Verification items for the finished model (mm, model axes). Face numbers are marked on the shaded views. A direction names the side the tool comes from. Give positions to 0.01 mm unless a question says otherwise; leave off trailing zeros. Loops run counter-clockwise (first coordinate to the right, second up) from the corner with the lowest first, then second, coordinate; pieces in that order, holes last. Notation, with made-up numbers: (78.5, -11) - (87.5, -11) arc R28 cw to (87.5, 19) - close; hole circle Ø2 at (-30, 0). An arc over 180 degrees is marked (long way). One line per item, written item: value. Start each with the question number.
1. Access from +Z, -Z, +X, -X, +Y, -Y to the whole of each face (thin tool, end or side, straight path). Record for the marked faces 5 and 6.
2. Sectioned sample at A-A (x = 0.75). Record the cut outline in (y, z), plus the area to 3 significant figures.
3. Scan lines: L1, parallel to Y at x = 1.5, z = -1.75; L2, parallel to Y at x = 6.75, z = -2; L3, parallel to Z at x = 5.5, y = -0.9. Record each from-to range of solid material in increasing order. Write a range as [from, to].
4. Gauge pin test, flat ends, axial feed: pin 1 (3 mm diameter, centred on x = 4.5, z = -3.5, fed in from -Y); pin 2 (2 mm diameter, centred on y = 1.5, z = -2.5, fed in from +X); pin 3 (1 mm diameter, centred on x = 3.5, y = -1, fed in from +Z). Record the tip position at first contact, or that the pin passes through.
5. Mould release check, pull along Z, two halves, no side actions. Record for the marked faces 1, 2, 3 and 4: pulls with the +Z half, pulls with the -Z half, needs draft (parallel to the pull), parting line crosses it, or undercut.
6. Sectioned sample at C-C (z = -6.75). Record the cut outline in (x, y).
7. Sectioned sample at B-B (y = 1.6). Record the cut outline in (x, z).
from build123d import *

# Parameters (mm, degrees)
SKETCH1_W               = 8
SKETCH1_H               = 8
BOSS_EXTRUDE1_DEPTH     = 3
CUT_EXTRUDE1_DEPTH      = 12.704699911
CUT_EXTRUDE1_DEPTH_BACK = 12.704699911
CUT_EXTRUDE2_DEPTH      = 11
SKETCH4_R               = 1.75
CUT_EXTRUDE3_DEPTH      = 0.4
SKETCH5_W               = 8
SKETCH5_H               = 1
BOSS_EXTRUDE2_DEPTH     = 2
FILLET1_R               = 4
CUT_EXTRUDE4_DEPTH      = 0.4
CUT_EXTRUDE5_DEPTH      = 0.5


with BuildPart() as part:
    # Sketch1 → Boss-Extrude1 (new body)
    with BuildSketch(Plane(origin=(0, 0, 0), x_dir=(1, 0, 0), z_dir=(0, 1, 0))):
        with Locations((4, 4)):
            Rectangle(SKETCH1_W, SKETCH1_H)
    extrude(amount=BOSS_EXTRUDE1_DEPTH)

    # Sketch2 → Cut-Extrude1 (cut, two sides: drawn at the far end of the back side and taken through both)
    with BuildSketch(Plane.XY.offset(-CUT_EXTRUDE1_DEPTH_BACK)):
        Polygon((0, 0), (0.6, 3), (0, 3), align=None)
        Polygon((8, 0), (7.4, 3), (8, 3), align=None)
    extrude(amount=CUT_EXTRUDE1_DEPTH + CUT_EXTRUDE1_DEPTH_BACK, mode=Mode.SUBTRACT)

    # Sketch3 → Cut-Extrude2 (cut)
    with BuildSketch(Plane(origin=(0, 0, 0), x_dir=(0, 0, -1), z_dir=(1, 0, 0))):
        Polygon((0, 0), (0.6, 3), (0, 3), align=None)
        Polygon((8, 3), (7.4, 3), (8, 0), align=None)
    extrude(amount=CUT_EXTRUDE2_DEPTH, mode=Mode.SUBTRACT)

    # Sketch4 → Cut-Extrude3 (cut)
    with BuildSketch(Plane.XZ):
        with Locations(Location((4, -3.75, 0), (0, 0, 270))):
            Circle(SKETCH4_R)
    extrude(amount=-CUT_EXTRUDE3_DEPTH, mode=Mode.SUBTRACT)

    # Sketch5 → Boss-Extrude2 (add)
    with BuildSketch(Plane.XZ):
        with Locations((4, -7.5)):
            Rectangle(SKETCH5_W, SKETCH5_H)
    extrude(amount=BOSS_EXTRUDE2_DEPTH)

    # Fillet1
    # the kernel refuses this fillet: 4 mm, written as the material it takes off along each edge
    with BuildSketch(Plane(origin=(8, -2, -16.660254038), x_dir=(0, 1, 0), z_dir=(0, 0, 1)), Plane(origin=(0, -2, 1.660254038), x_dir=(0, 1, 0), z_dir=(0, 0, -1))) as fillet1_piece_1:
        with BuildLine():
            CenterArc((4, 3.464101615), FILLET1_R, 180, 60)
            Line((0, 3.464101615), (-0.08, 3.464101615))
            Line((-0.08, 3.464101615), (-0.08, 0))
            Line((-0.08, 0), (0, -0.08))
            ThreePointArc((0, -0.08), (1, -0.08), (1.96, -0.069282032))
            Line((1.96, -0.069282032), (2, 0))
        make_face()
    extrude(amount=18.320508076, mode=Mode.SUBTRACT)

    # Sketch6 → Cut-Extrude4 (cut)
    with BuildSketch(Plane(origin=(0, 3, 0), x_dir=(1, 0, 0), z_dir=(0, 1, 0))):
        with BuildLine():
            add(Edge.make_bspline(
                [(5.284087955, 2.773445367), (5.333545491, 2.739545524), (5.432652736, 2.671614118), (5.590291823, 2.583736248), (5.752942084, 2.503846486), (5.865979951, 2.460876102), (5.92270975, 2.439310751)],
                knots=[0, 0, 0, 0, 0.994855506, 1.99357661, 2.993045438, 4, 4, 4, 4], degree=3))
            Line((5.92270975, 2.439310751), (5.628639237, 1.875208187))
            add(Edge.make_bspline(
                [(5.628639237, 1.875208187), (5.568520037, 1.893818156), (5.447325875, 1.93133395), (5.332925255, 1.986187111), (5.275273852, 2.013829982)],
                knots=[0, 0, 0, 0, 0.992113803, 2, 2, 2, 2], degree=3))
            add(Edge.make_bspline(
                [(5.275273852, 2.013829982), (5.26961656, 2.016684314), (5.253233801, 2.024950075), (5.223476786, 2.045298413), (5.178074812, 2.072724498), (5.118973761, 2.11071311), (5.045578888, 2.157800121), (4.95765273, 2.213934729), (4.856407872, 2.280704114), (4.783596416, 2.327731001), (4.744825134, 2.35277229)],
                knots=[0, 0, 0, 0, 0.241377655, 0.698997227, 1.371388316, 2.263975901, 3.376788369, 4.695767198, 6.240533187, 8, 8, 8, 8], degree=3))
            add(Edge.make_bspline(
                [(4.744825134, 2.35277229), (4.712670389, 2.339001865), (4.648050063, 2.311327899), (4.547788838, 2.27725121), (4.444978029, 2.248544986), (4.339982896, 2.224200245), (4.232359046, 2.206111381), (4.122258624, 2.192239309), (4.00937299, 2.18410397), (3.933139287, 2.183304154), (3.894664878, 2.182900495)],
                knots=[0, 0, 0, 0, 0.961025642, 1.931341354, 2.907359807, 3.893838693, 4.891829695, 5.905170566, 6.942759923, 8, 8, 8, 8], degree=3))
            add(Edge.make_bspline(
                [(3.894664878, 2.182900495), (3.821683976, 2.184676763), (3.679027131, 2.188148859), (3.471015208, 2.212756542), (3.275562804, 2.255408477), (3.091812023, 2.313667662), (2.920867424, 2.390147666), (2.761229426, 2.482594503), (2.615108223, 2.593406711), (2.480490537, 2.71918809), (2.361392609, 2.861354588), (2.257130725, 3.017424584), (2.168806746, 3.186880722), (2.097587685, 3.370615377), (2.041301668, 3.567142879), (2.002926315, 3.777850586), (1.978227581, 4.001488849), (1.975427333, 4.155321196), (1.973991801, 4.234182546)],
                knots=[0, 0, 0, 0, 1.098101164, 2.146474535, 3.146072545, 4.104420533, 5.041773038, 5.958565538, 6.874115049, 7.795336865, 8.725215067, 9.658214839, 10.614563411, 11.594512188, 12.618591104, 13.685899083, 14.813688224, 16, 16, 16, 16], degree=3))
            add(Edge.make_bspline(
                [(1.973991801, 4.234182546), (1.97543059, 4.313040679), (1.978227497, 4.466335509), (2.002757559, 4.689542909), (2.042412611, 4.899497801), (2.098124704, 5.096337583), (2.170410456, 5.279545107), (2.259079723, 5.449017762), (2.363505524, 5.605417057), (2.484015277, 5.747270094), (2.617919267, 5.874338646), (2.764464989, 5.984327234), (2.9219486, 6.078236158), (3.090996271, 6.154643933), (3.272074664, 6.212871015), (3.463805003, 6.255387163), (3.667248709, 6.280295733), (3.806454886, 6.283712517), (3.877837955, 6.285464598)],
                knots=[0, 0, 0, 0, 1.193283781, 2.319662245, 3.393996131, 4.424093603, 5.411284417, 6.369670503, 7.313761776, 8.251713527, 9.181123148, 10.102053383, 11.01932051, 11.951118596, 12.903560284, 13.893239571, 14.919681386, 16, 16, 16, 16], degree=3))
            add(Edge.make_bspline(
                [(3.877837955, 6.285464598), (3.948708316, 6.284176334), (4.086935049, 6.281663683), (4.288489067, 6.254790298), (4.478939684, 6.214016744), (4.658513444, 6.155241629), (4.826290277, 6.078911265), (4.983143341, 5.98623667), (5.128157857, 5.876434989), (5.26137487, 5.750578969), (5.380523981, 5.609215368), (5.486073462, 5.454669187), (5.572731816, 5.285035211), (5.645736122, 5.103191508), (5.700157026, 4.90736457), (5.740330715, 4.69867705), (5.764520815, 4.476471411), (5.76739165, 4.323719862), (5.768863596, 4.245400495)],
                knots=[0, 0, 0, 0, 1.078752742, 2.104017338, 3.091035458, 4.041673215, 4.975566109, 5.892967701, 6.810684895, 7.740128604, 8.678185021, 9.621404646, 10.583875016, 11.573429805, 12.6009998, 13.674031063, 14.80742018, 16, 16, 16, 16], degree=3))
            add(Edge.make_bspline(
                [(5.768863596, 4.245400495), (5.767275795, 4.16278925), (5.764189157, 4.002195454), (5.737326284, 3.768977018), (5.693780668, 3.550562854), (5.648918616, 3.41330904), (5.627036673, 3.346362034)],
                knots=[0, 0, 0, 0, 1.083667057, 2.106616435, 3.076482036, 4, 4, 4, 4], degree=3))
            add(Edge.make_bspline(
                [(5.627036673, 3.346362034), (5.607421404, 3.297050064), (5.567517691, 3.196733787), (5.488642668, 3.051933408), (5.394797316, 2.909076479), (5.321514211, 2.819296637), (5.284087955, 2.773445367)],
                knots=[0, 0, 0, 0, 0.948216854, 1.928975575, 2.942311585, 4, 4, 4, 4], degree=3))
        make_face()
        with BuildLine():
            add(Edge.make_bspline(
                [(4.642261032, 3.185304341), (4.671182259, 3.216922768), (4.72909393, 3.280235293), (4.800707281, 3.388678336), (4.863230922, 3.50497094), (4.912388312, 3.632014464), (4.951923574, 3.76787431), (4.97951585, 3.913560578), (4.996652709, 4.068707035), (4.998621406, 4.175375245), (4.999632827, 4.230176136)],
                knots=[0, 0, 0, 0, 0.906820982, 1.815812261, 2.745108282, 3.70056618, 4.696560745, 5.740060838, 6.83895416, 8, 8, 8, 8], degree=3))
            add(Edge.make_bspline(
                [(4.999632827, 4.230176136), (4.998745764, 4.286560817), (4.997027382, 4.395786947), (4.982794262, 4.554398979), (4.957747484, 4.70183414), (4.925058455, 4.838707416), (4.88052022, 4.963910999), (4.826807351, 5.078388614), (4.763835344, 5.182421929), (4.690056733, 5.274294514), (4.608907177, 5.355063587), (4.522159409, 5.426414517), (4.428546166, 5.486139657), (4.328544236, 5.534184829), (4.222990468, 5.571989212), (4.111634776, 5.59943433), (3.994225982, 5.615495039), (3.913944994, 5.6176829), (3.873030263, 5.618797931)],
                knots=[0, 0, 0, 0, 1.335693338, 2.587451293, 3.768164612, 4.876224393, 5.916940853, 6.910477009, 7.867661778, 8.790666633, 9.694493319, 10.576027549, 11.446684429, 12.318352473, 13.199023277, 14.098364444, 15.030842682, 16, 16, 16, 16], degree=3))
            add(Edge.make_bspline(
                [(3.873030263, 5.618797931), (3.831841607, 5.617719084), (3.751279942, 5.615608947), (3.633755604, 5.599158788), (3.522145798, 5.573035665), (3.416723766, 5.534932642), (3.316536446, 5.486796326), (3.222573421, 5.427181815), (3.134847786, 5.356951252), (3.053289548, 5.276692152), (2.980446173, 5.184790487), (2.915694165, 5.082568667), (2.862164439, 4.968850144), (2.819178201, 4.84427298), (2.784825228, 4.709477379), (2.760087026, 4.563739976), (2.745835322, 4.407279692), (2.744110931, 4.299383286), (2.74322257, 4.243797931)],
                knots=[0, 0, 0, 0, 0.980107447, 1.917010591, 2.819119613, 3.703969481, 4.579773866, 5.459928929, 6.346604172, 7.250235365, 8.177620171, 9.131899985, 10.124404622, 11.161948974, 12.264485933, 13.431998172, 14.677033863, 16, 16, 16, 16], degree=3))
            add(Edge.make_bspline(
                [(2.74322257, 4.243797931), (2.744089067, 4.187408458), (2.745771696, 4.077907007), (2.760333697, 3.91913972), (2.783941374, 3.771215716), (2.817547327, 3.634196218), (2.86051391, 3.507924697), (2.913437174, 3.392577112), (2.976036542, 3.288297709), (3.048513511, 3.196032652), (3.128245057, 3.114861766), (3.213441608, 3.04409835), (3.303411645, 2.983479498), (3.39857486, 2.934226809), (3.498956775, 2.896402137), (3.604207339, 2.869103357), (3.714939061, 2.852831885), (3.790443662, 2.850669982), (3.82895975, 2.849567162)],
                knots=[0, 0, 0, 0, 1.356840463, 2.634818045, 3.833173645, 4.958776583, 6.025986406, 7.038359119, 8.007356852, 8.946032033, 9.855123386, 10.740685277, 11.607120956, 12.460971081, 13.313368256, 14.183325659, 15.073285775, 16, 16, 16, 16], degree=3))
            add(Edge.make_bspline(
                [(3.82895975, 2.849567162), (3.857844622, 2.850073951), (3.914741814, 2.851072222), (3.998801079, 2.862293633), (4.080683558, 2.878515583), (4.133570622, 2.895033243), (4.159889237, 2.903253059)],
                knots=[0, 0, 0, 0, 1.028828871, 2.026578908, 3.017950568, 4, 4, 4, 4], degree=3))
            add(Edge.make_bspline(
                [(4.159889237, 2.903253059), (4.119539232, 2.924336443), (4.039635796, 2.966086993), (3.916101198, 3.019284802), (3.792319766, 3.067214804), (3.708133251, 3.09310976), (3.666299493, 3.105977418)],
                knots=[0, 0, 0, 0, 1.021704821, 2.023239566, 3.017713044, 4, 4, 4, 4], degree=3))
            Line((3.666299493, 3.105977418), (3.889857186, 3.56751588))
            add(Edge.make_bspline(
                [(3.889857186, 3.56751588), (3.955233958, 3.544923565), (4.086618506, 3.49952088), (4.276409331, 3.409366748), (4.463555304, 3.306758821), (4.582244486, 3.226093623), (4.642261032, 3.185304341)],
                knots=[0, 0, 0, 0, 0.979271047, 1.967993817, 2.972492781, 4, 4, 4, 4], degree=3))
        make_face(mode=Mode.SUBTRACT)
    extrude(amount=-CUT_EXTRUDE4_DEPTH, mode=Mode.SUBTRACT)

    # Sketch7 → Cut-Extrude5 (cut)
    with BuildSketch(Plane(origin=(0, 3, 0), x_dir=(1, 0, 0), z_dir=(0, 1, 0))):
        with BuildLine():
            Line((6.989609495, 0.992731968), (6.662686419, 0.992731968))
            Line((6.662686419, 0.992731968), (6.662686419, 2.203028442))
            add(Edge.make_bspline(
                [(6.662686419, 2.203028442), (6.647868508, 2.187985499), (6.618433709, 2.158103687), (6.571421698, 2.116422543), (6.522616062, 2.07764809), (6.471533827, 2.042148614), (6.418842766, 2.009418309), (6.364004407, 1.979715431), (6.307416238, 1.952628999), (6.268215163, 1.937491891), (6.248583854, 1.929911455)],
                knots=[0, 0, 0, 0, 1.012567276, 2.011397996, 3.011400399, 4.000747768, 4.993445519, 5.985067596, 6.990952157, 8, 8, 8, 8], degree=3))
            Line((6.248583854, 1.929911455), (6.248583854, 2.256834532))
            add(Edge.make_bspline(
                [(6.248583854, 2.256834532), (6.270355964, 2.264998139), (6.315923296, 2.282083933), (6.383165354, 2.318426283), (6.453350876, 2.363421778), (6.512310721, 2.40755194), (6.559122414, 2.44678718), (6.591840229, 2.478326157), (6.622155165, 2.510623705), (6.648927745, 2.544722271), (6.672860762, 2.579932457), (6.694066458, 2.616196741), (6.712732345, 2.65362968), (6.722503807, 2.679697149), (6.727389944, 2.692731968)],
                knots=[0, 0, 0, 0, 1.253673617, 2.623841347, 4.114270668, 5.751233548, 6.594491912, 7.409089316, 8.202422231, 8.983165545, 9.746111525, 10.498431446, 11.249153235, 12, 12, 12, 12], degree=3))
            Line((6.727389944, 2.692731968), (6.989609495, 2.692731968))
            Line((6.989609495, 2.692731968), (6.989609495, 0.992731968))
        make_face()
    extrude(amount=-CUT_EXTRUDE5_DEPTH, mode=Mode.SUBTRACT)


solid = part.part
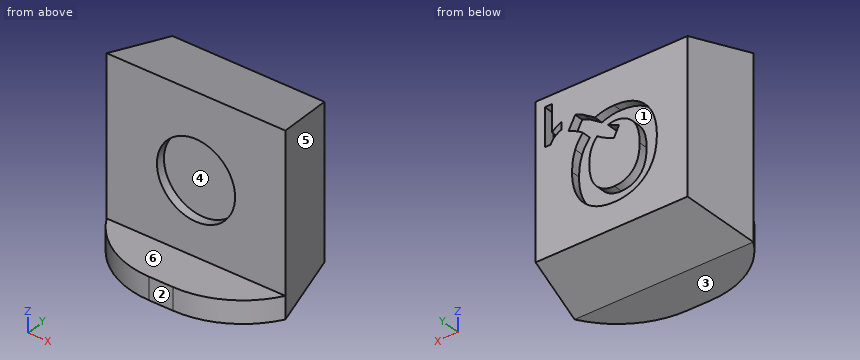
Results are:
1. face 5: +Z, -Z, +X, +Y
1. face 6: +Z, +X, -X, -Y
2. outline: (-0.94, -8) - (0, -8) - (3, -7.4) - (3, -0.6) - (0, 0) - (0, -7) - (-0.94, -7) - close
2. area: 23.1 mm^2
3. L1: y = [0, 3]
3. L2: y = [0, 2.5]
3. L3: z = [-8, -7]
4. pin 1: stops at y = 0
4. pin 2: stops at x = 7.9
4. pin 3: stops at z = -7
5. face 1: undercut
5. face 2: needs draft
5. face 3: pulls with the -Z half
5. face 4: undercut
6. outline: (0, 0) - (8, 0) - (7.4, 3) - (0.6, 3) - close
7. outline: (0.32, -7.68) - (7.68, -7.68) - (7.68, -0.32) - (0.32, -0.32) - close
